```python
from build123d import *

# Parameters (mm, degrees)
F0_R     = 4.5
F1_DEPTH = 3
F2_SIZE2 = 2.99999
F2_SIZE  = 2.99999


# Not quite as in the source:
# - a fillet or chamfer is up to 0.001 mm smaller than in the source, because OpenCascade refuses the exact size


with BuildPart() as f1:
    # F0 (on Top) → F1 (new body)
    with BuildSketch(Plane.XY):
        with BuildLine():
            ThreePointArc((12.0512473873, -8.9312617479), (14.2437479409, -4.7027273571), (15, 0))
            ThreePointArc((15, 0), (14.9998319689, 0.07099932), (14.9993278795, 0.1419970492))
            Line((14.9993278795, 0.1419970492), (9.794719653, -1.5490826747))
            Line((9.794719653, -1.5490826747), (7.0135667036, 7.0104259719))
            Line((7.0135667036, 7.0104259719), (12.2181749302, 8.7015056959))
            ThreePointArc((12.2181749302, 8.7015056959), (8.8167787844, 12.1352549156), (4.5, 14.3090880213))
            Line((4.5, 14.3090880213), (4.5, 8.8366390791))
            Line((4.5, 8.8366390791), (-4.5, 8.8366390791))
            Line((-4.5, 8.8366390791), (-4.5, 14.3090880213))
            ThreePointArc((-4.5, 14.3090880213), (-8.8167787844, 12.1352549156), (-12.2181749302, 8.7015056959))
            Line((-12.2181749302, 8.7015056959), (-7.0135667036, 7.0104259719))
            Line((-7.0135667036, 7.0104259719), (-9.794719653, -1.5490826747))
            Line((-9.794719653, -1.5490826747), (-14.9993278795, 0.1419970492))
            ThreePointArc((-14.9993278795, 0.1419970492), (-14.2658477444, -4.6352549156), (-12.0512473873, -8.9312617479))
            Line((-12.0512473873, -8.9312617479), (-8.8346226052, -4.5039575528))
            Line((-8.8346226052, -4.5039575528), (-1.5534696558, -9.7940248235))
            Line((-1.5534696558, -9.7940248235), (-4.770094438, -14.2213290185))
            ThreePointArc((-4.770094438, -14.2213290185), (0, -15), (4.770094438, -14.2213290185))
            Line((4.770094438, -14.2213290185), (1.5534696558, -9.7940248235))
            Line((1.5534696558, -9.7940248235), (8.8346226052, -4.5039575528))
            Line((8.8346226052, -4.5039575528), (12.0512473873, -8.9312617479))
        make_face()
        Circle(F0_R, mode=Mode.SUBTRACT)
        with BuildLine():
            Line((9.794719653, -1.5490826747), (14.9993278795, 0.1419970492))
            ThreePointArc((14.9993278795, 0.1419970492), (14.2658477444, 4.6352549156), (12.2181749302, 8.7015056959))
            Line((12.2181749302, 8.7015056959), (7.0135667036, 7.0104259719))
            Line((7.0135667036, 7.0104259719), (9.794719653, -1.5490826747))
        make_face()
        with BuildLine():
            ThreePointArc((12.2181749302, 8.7015056959), (14.2658477444, 4.6352549156), (14.9993278795, 0.1419970492))
            Line((14.9993278795, 0.1419970492), (25.1669893821, 3.445670536))
            Line((25.1669893821, 3.445670536), (22.3858364327, 12.0051791827))
            Line((22.3858364327, 12.0051791827), (12.2181749302, 8.7015056959))
        make_face()
        with BuildLine():
            Line((18.335207782, -17.5803912241), (12.0512473873, -8.9312617479))
            ThreePointArc((12.0512473873, -8.9312617479), (8.8167787844, -12.1352549156), (4.770094438, -14.2213290185))
            Line((4.770094438, -14.2213290185), (11.0540548326, -22.8704584947))
            Line((11.0540548326, -22.8704584947), (18.335207782, -17.5803912241))
        make_face()
        with BuildLine():
            ThreePointArc((4.770094438, -14.2213290185), (8.8167787844, -12.1352549156), (12.0512473873, -8.9312617479))
            Line((12.0512473873, -8.9312617479), (8.8346226052, -4.5039575528))
            Line((8.8346226052, -4.5039575528), (1.5534696558, -9.7940248235))
            Line((1.5534696558, -9.7940248235), (4.770094438, -14.2213290185))
        make_face()
        Polygon((22.3858364327, 12.0051791827), (25.1669893821, 3.445670536), (26.8665828511, -1.7851403036), (38.0422606518, 12.360679775), (20.6862429636, 17.2359900223), align=None)
        Polygon((22.7848012511, -14.3475723364), (18.335207782, -17.5803912241), (11.0540548326, -22.8704584947), (6.6044613636, -26.1032773823), (23.5114100917, -32.360679775), align=None)
        with BuildLine():
            Line((4.5, 8.8366390791), (4.5, 14.3090880213))
            ThreePointArc((4.5, 14.3090880213), (0, 15), (-4.5, 14.3090880213))
            Line((-4.5, 14.3090880213), (-4.5, 8.8366390791))
            Line((-4.5, 8.8366390791), (4.5, 8.8366390791))
        make_face()
        with BuildLine():
            ThreePointArc((-4.5, 14.3090880213), (0, 15), (4.5, 14.3090880213))
            Line((4.5, 14.3090880213), (4.5, 25))
            Line((4.5, 25), (-4.5, 25))
            Line((-4.5, 25), (-4.5, 14.3090880213))
        make_face()
        with BuildLine():
            Line((-11.0540548326, -22.8704584947), (-4.770094438, -14.2213290185))
            ThreePointArc((-4.770094438, -14.2213290185), (-8.8167787844, -12.1352549156), (-12.0512473873, -8.9312617479))
            Line((-12.0512473873, -8.9312617479), (-18.335207782, -17.5803912241))
            Line((-18.335207782, -17.5803912241), (-11.0540548326, -22.8704584947))
        make_face()
        with BuildLine():
            ThreePointArc((-12.0512473873, -8.9312617479), (-8.8167787844, -12.1352549156), (-4.770094438, -14.2213290185))
            Line((-4.770094438, -14.2213290185), (-1.5534696558, -9.7940248235))
            Line((-1.5534696558, -9.7940248235), (-8.8346226052, -4.5039575528))
            Line((-8.8346226052, -4.5039575528), (-12.0512473873, -8.9312617479))
        make_face()
        Polygon((-4.5, 25), (4.5, 25), (10, 25), (0, 40), (-10, 25), align=None)
        Polygon((-6.6044613636, -26.1032773823), (-11.0540548326, -22.8704584947), (-18.335207782, -17.5803912241), (-22.7848012511, -14.3475723364), (-23.5114100917, -32.360679775), align=None)
        with BuildLine():
            Line((-7.0135667036, 7.0104259719), (-12.2181749302, 8.7015056959))
            ThreePointArc((-12.2181749302, 8.7015056959), (-14.2658477444, 4.6352549156), (-14.9993278795, 0.1419970492))
            Line((-14.9993278795, 0.1419970492), (-9.794719653, -1.5490826747))
            Line((-9.794719653, -1.5490826747), (-7.0135667036, 7.0104259719))
        make_face()
        with BuildLine():
            ThreePointArc((-14.9993278795, 0.1419970492), (-14.2658477444, 4.6352549156), (-12.2181749302, 8.7015056959))
            Line((-12.2181749302, 8.7015056959), (-22.3858364327, 12.0051791827))
            Line((-22.3858364327, 12.0051791827), (-25.1669893821, 3.445670536))
            Line((-25.1669893821, 3.445670536), (-14.9993278795, 0.1419970492))
        make_face()
        Polygon((-25.1669893821, 3.445670536), (-22.3858364327, 12.0051791827), (-20.6862429636, 17.2359900223), (-38.0422606518, 12.360679775), (-26.8665828511, -1.7851403036), align=None)
    extrude(amount=F1_DEPTH)

    # F2 (size 3 and 3 in the source; OpenCascade refuses exactly that, so slightly less here)
    f2_edges = [f1.edges().sort_by_distance(p)[0] for p in [
        (-15.193228, -13.255826, 3),
        (-20.560005, -15.963982, 3),
        (-23.148106, -23.354126, 3),
        (-15.057936, -29.231979, 3),
        (-8.829258, -24.486868, 3),
        (-7.912075, -18.545894, 3),
        (0, -15, 3),
        (7.912075, -18.545894, 3),
        (8.829258, -24.486868, 3),
        (15.057936, -29.231979, 3),
        (23.148106, -23.354126, 3),
        (20.560005, -15.963982, 3),
        (15.193228, -13.255826, 3),
        (14.265848, -4.635255, 3),
        (20.083159, 1.793834, 3),
        (26.016786, 0.830265, 3),
        (32.454422, 5.28777, 3),
        (29.364252, 14.798335, 3),
        (21.53604, 14.620585, 3),
        (17.302006, 10.353342, 3),
        (8.816779, 12.135255, 3),
        (4.5, 19.654544, 3),
        (7.25, 25, 3),
        (5, 32.5, 3),
        (-5, 32.5, 3),
        (-7.25, 25, 3),
        (-4.5, 19.654544, 3),
        (-8.816779, 12.135255, 3),
        (-17.302006, 10.353342, 3),
        (-21.53604, 14.620585, 3),
        (-29.364252, 14.798335, 3),
        (-32.454422, 5.28777, 3),
        (-26.016786, 0.830265, 3),
        (-20.083159, 1.793834, 3),
        (-14.265848, -4.635255, 3),
        (-4.5, 0, 3),
    ]]
    chamfer(f2_edges, length=F2_SIZE, length2=F2_SIZE2)


solid = f1.part
```
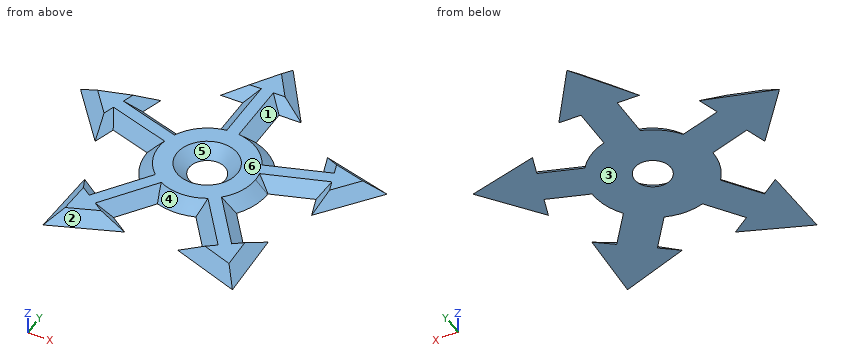
CAD build for the part. Positions are in the model's coordinates, mm. Face numbers are marked on the shaded views. A direction names the side the tool comes from. Round coordinates to 2 decimals unless told otherwise and drop trailing zeros. Return JSON: item names as keys, results as strings. Group by question number.
(1) Drop flat-ended pins along their axis: P1, Ø1, axis at x = -10.5, z = 1, coming from the -Y side; P2, Ø3, axis at x = -12.5, y = -8, coming from the -Z side; P3, Ø4, axis at x = -18.5, y = 14, coming from the -Z side (1 decimal); P4, Ø1.5, axis at y = -9.5, z = 1.5, coming from the +X side. Give the stop position or say it passes through.
(2) Wall check: probe 1 along X at (y, z) = (-19, 1.95); probe 2 along X at (y, z) = (-11, 2.85); probe 3 along X at (y, z) = (0, 0.05). Give the ranges that are in metal, low to high. Write a range as [from, to].
(3) Saw through at A-A, the plane y = 1. Give the number of separate pieces and of enclosed holes in the cut face, and give its area (3 significant figures).
(4) Mould opens along Y. For the marked faces 4, 5 and 6 say: +Y half, -Y half, draft (parallel to the pull), parting line (faces both ways), or undercut.
(5) Tool access for the marked faces 1, 2 and 3: list every direction of +Z, -Z, +X, -X, +Y, -Y with a clear straight run to the whole face (end or side of a thin tool).
Answer list:
{
 "1": {"P1": "y = -27.04", "P2": "z = 0", "P3": "through", "P4": "x = 11.69"},
 "2": {"probe 1": "[-21.02, -19.7], [-16.96, -10.65], [10.65, 16.96], [19.7, 21.02]", "probe 2": "[-10.03, -5.95], [-5.16, 5.16], [5.95, 10.03]", "probe 3": "[-28.21, -26.34], [-14.95, -4.55], [4.55, 14.95], [26.34, 28.21]"},
 "3": {"separate pieces": "4", "enclosed holes": "0", "area": "52.6 mm2"},
 "4": {"face 4": "-Y half", "face 5": "undercut", "face 6": "draft"},
 "5": {"face 1": "+Z", "face 2": "+Z, -Y", "face 3": "-Z, +X, -X, +Y, -Y"}
}
